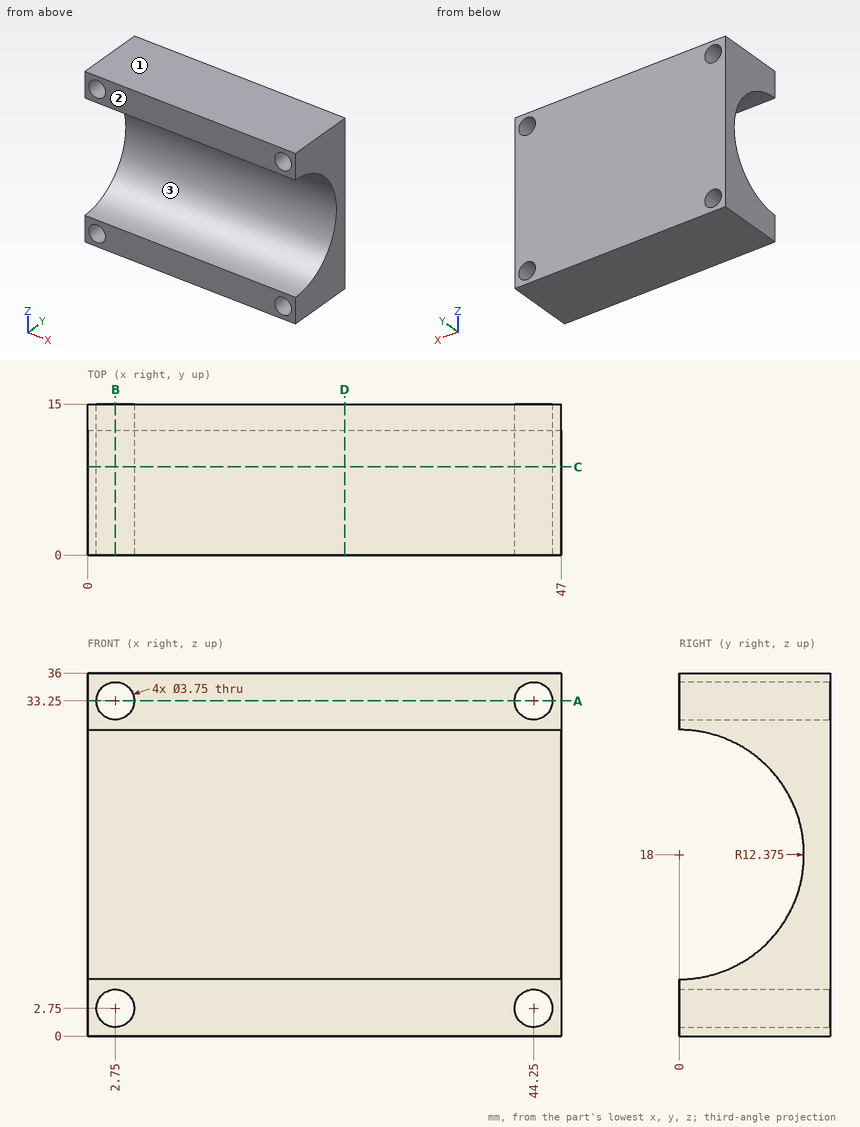
For this review, use the dimensioned drawing (mm, ordinates from the lowest corner) and the shaded views. Give positions to 0.01 mm unless a question says otherwise; leave off trailing zeros. Order: outer loops, then holes, each group sorted by start corner. A loop starts at its lowest first (then second) coordinate and runs counter-clockwise, first axis right, second up. Notation, with made-up numbers: (24.25, 21.5) - (40.25, 21.5) arc R8 ccw to (40.25, 33.5) - close; hole circle Ø1 at (38, -2). An arc over 180 degrees is marked (long way). Write item = value, one per line. Start each with the question number.
Q1. We need section A-A on z = 33.25. State the section outline as (x, y) points (3 decimals).
Q2. We need section B-B on x = 2.75. State the section outline as (y, z) points (3 decimals), plus the area to 3 significant figures.
Q3. Clearance check with a flat-ended pin moving along its axis: pin 1 Ø6 at (x, z) = (2.75, 2.75) entering from +Y. State where the tip first meets the part, or that it passes through.
Q4. To check wall thickness, follow L1, parallel to X at y = 6, z = 2.75 (3 decimals); L2, parallel to Z at x = 2.75, y = 8.75 (3 decimals); L3, parallel to Z at x = 2.75, y = 3.75 (3 decimals). State the ranges of each line that lie inside material, in increasing order. Write a range as from..to.
Q5. Mouldability with a two-part tool opening along Z and no side actions: class the marked faces 1, 2 and 3 as released by +Z, released by -Z, zero draft, split by the parting line, or undercut.
Q6. We need section D-D on x = 25.5. State the section outline as (y, z) points (3 decimals).
Q7. We need section C-C on y = 8.75. State the section outline as (x, z) points (3 decimals), plus the area to 3 significant figures.
Working result:
q1.outline = (0, 0) - (0.875, 0) - (0.875, 15) - (0, 15) - close; (4.625, 0) - (42.375, 0) - (42.375, 15) - (4.625, 15) - close; (46.125, 0) - (47, 0) - (47, 15) - (46.125, 15) - close
q2.outline = (0, 0) - (15, 0) - (15, 0.875) - (0, 0.875) - close; (0, 4.625) - (15, 4.625) - (15, 31.375) - (0, 31.375) - (0, 30.375) arc R12.375 cw to (0, 5.625) - close; (0, 35.125) - (15, 35.125) - (15, 36) - (0, 36) - close
q2.area = 187 mm²
q3.pin_1 = 15
q4.L1 = 0..0.875, 4.625..42.375, 46.125..47
q4.L2 = 0..0.875, 4.625..9.249, 26.751..31.375, 35.125..36
q4.L3 = 0..0.875, 4.625..6.207, 29.793..31.375, 35.125..36
q5.face_1 = released by +Z
q5.face_2 = zero draft
q5.face_3 = undercut
q6.outline = (0, 0) - (15, 0) - (15, 36) - (0, 36) - (0, 30.375) arc R12.375 cw to (0, 5.625) - close
q7.outline = (0, 0) - (47, 0) - (47, 9.249) - (0, 9.249) - close; (0, 26.751) - (47, 26.751) - (47, 36) - (0, 36) - close; hole circle Ø3.75 at (2.75, 2.75); hole circle Ø3.75 at (2.75, 33.25); hole circle Ø3.75 at (44.25, 2.75); hole circle Ø3.75 at (44.25, 33.25)
q7.area = 825 mm²
